Source: CAD feature listing. Evaluate the final solid. Frame: model axes, mm. Face numbers are marked on the shaded views. A direction names the side the tool comes from. Give positions to 0.01 mm unless a question says otherwise; leave off trailing zeros. Loops run counter-clockwise (first coordinate to the right, second up) from the corner with the lowest first, then second, coordinate; pieces in that order, holes last.
```python
from build123d import *

# Parameters (mm, degrees)
SKETCH_234_R           = 1.55
EXTRUDE_1_DEPTH        = 2.75
SKETCH_923_W           = 10.000000002
SKETCH_923_H           = 4.75
EXTRUDE_2_DEPTH        = 2.75
SKETCH_1070_W          = 1
SKETCH_1070_H          = 6.95
EXTRUDE_1769_DEPTH     = 2.75
PCB_START              = -4
SKETCH_6_W             = 1
SKETCH_6_H             = 6.95
PCB_DEPTH              = 4
SKETCH_4_W             = 1.75
SKETCH_4_H             = 28.99988509
CUT_EXTRUDE_2211_DEPTH = 1.5
SKETCH_5_W             = 0.25
SKETCH_5_H             = 28.99988509
CUT_EXTRUDE_2_DEPTH    = 33.350081892
CHAMFER_1_SIZE         = 1
CHAMFER_2_SIZE         = 1
CUT_EXTRUDE_4_DEPTH    = 4


with BuildPart() as part:
    # Sketch 234 → 底座-1 (new body)
    with BuildSketch(Plane(origin=(0, 0, 0), x_dir=(1, 0, 0), z_dir=(0, 1, 0))):
        with BuildLine():
            Line((22.500000002, -14.24988509), (22.500000002, -7.263629174))
            Line((22.500000002, -7.263629174), (24.500000002, -7.263629174))
            Line((24.500000002, -7.263629174), (24.500000002, 0.312480077))
            Line((24.500000002, 0.312480077), (24.715186194, 2.08073674))
            ThreePointArc((24.715186194, 2.08073674), (20.15501929, 5.688743466), (16.252981126, 10))
            Line((16.252981126, 10), (12.5, 10))
            Line((12.5, 10), (12.5, -14.24988509))
            Line((12.5, -14.24988509), (22.500000002, -14.24988509))
        make_face()
        with Locations(Location((16.865979255, 0, 0), (0, 0, 270))):
            Circle(SKETCH_234_R, mode=Mode.SUBTRACT)
    extrude(amount=EXTRUDE_1_DEPTH)

    # Sketch 923 → 底座-2 (add)
    with BuildSketch(Plane(origin=(0, 0, 0), x_dir=(1, 0, 0), z_dir=(0, 1, 0))):
        with Locations((17.500000001, -16.62488509)):
            Rectangle(SKETCH_923_W, SKETCH_923_H)
    extrude(amount=EXTRUDE_2_DEPTH)

    # Sketch 1070 → Extrude 1769 (add)
    with BuildSketch(Plane(origin=(0, 0, 0), x_dir=(1, 0, 0), z_dir=(0, 1, 0))):
        with BuildLine():
            ThreePointArc((24.715186194, 2.08073674), (25.291636518, 1.705823535), (25.875319612, 1.342273079))
            Line((25.875319612, 1.342273079), (25.750000002, 0.312480077))
            Line((25.750000002, 0.312480077), (25.750000002, -14.213629174))
            Line((25.750000002, -14.213629174), (24.500000002, -14.213629174))
            Line((24.500000002, -14.213629174), (24.500000002, -7.263629174))
            Line((24.500000002, -7.263629174), (24.500000002, 0.312480077))
            Line((24.500000002, 0.312480077), (24.715186194, 2.08073674))
        make_face()
        with Locations((24.000000002, -10.738629174)):
            Rectangle(SKETCH_1070_W, SKETCH_1070_H)
        with Locations((23.000000002, -10.738629174)):
            Rectangle(SKETCH_1070_W, SKETCH_1070_H)
    extrude(amount=EXTRUDE_1769_DEPTH)

    # Sketch 6 → 底座卡榫-注意PCB突出部分 (add)
    with BuildSketch(Plane(origin=(0, 0, 0), x_dir=(1, 0, 0), z_dir=(0, 1, 0)).offset(PCB_START)):
        with Locations((24.000000002, -10.738629174)):
            Rectangle(SKETCH_6_W, SKETCH_6_H)
        with BuildLine():
            ThreePointArc((24.715186194, 2.08073674), (25.291636518, 1.705823535), (25.875319612, 1.342273079))
            Line((25.875319612, 1.342273079), (25.750000002, 0.312480077))
            Line((25.750000002, 0.312480077), (25.750000002, -14.213629174))
            Line((25.750000002, -14.213629174), (24.500000002, -14.213629174))
            Line((24.500000002, -14.213629174), (24.500000002, -7.263629174))
            Line((24.500000002, -7.263629174), (24.500000002, 0.312480077))
            Line((24.500000002, 0.312480077), (24.715186194, 2.08073674))
        make_face()
    extrude(amount=PCB_DEPTH)

    # 草图4 → Cut-Extrude 2211 (cut)
    with BuildSketch(Plane(origin=(0, 0, 0), x_dir=(1, 0, 0), z_dir=(0, 1, 0))):
        with Locations((13.375, -4.499942545)):
            Rectangle(SKETCH_4_W, SKETCH_4_H)
    extrude(amount=CUT_EXTRUDE_2211_DEPTH, mode=Mode.SUBTRACT)

    # 草图5 → 配合切除-2 (cut, through all)
    with BuildSketch(Plane(origin=(0, 0, 0), x_dir=(1, 0, 0), z_dir=(0, 1, 0))):
        with Locations((12.625, -4.499942545)):
            Rectangle(SKETCH_5_W, SKETCH_5_H)
    extrude(amount=CUT_EXTRUDE_2_DEPTH, mode=Mode.SUBTRACT)

    # 倒角1
    chamfer_1_edges = [part.edges().sort_by_distance(p)[0] for p in [
        (22.500000002, 1.375, 18.99988509),
        (20.661675073, 2.75, -5.223818951),
        (22.500000002, 1.375, 14.213629174),
    ]]
    chamfer(chamfer_1_edges, length=CHAMFER_1_SIZE)

    # 倒角2
    chamfer_2_edges = [part.edges().sort_by_distance(p)[0] for p in [
        (16.865979255, 2.75, -1.55),
    ]]
    chamfer(chamfer_2_edges, length=CHAMFER_2_SIZE)

    # Sketch 6 2 → 切除-拉伸4 (cut)
    with BuildSketch(Plane.XZ.offset(4)):
        with BuildLine():
            Line((24.715186194, -2.08073674), (24.500000002, -0.312480077))
            Line((24.500000002, -0.312480077), (24.500000002, 7.263629174))
            Line((24.500000002, 7.263629174), (23.500000002, 7.263629174))
            Line((23.500000002, 7.263629174), (23.500000002, 7.513629174))
            Line((23.500000002, 7.513629174), (24.750000002, 7.513629174))
            Line((24.750000002, 7.513629174), (24.750000002, -0.312480077))
            Line((24.750000002, -0.312480077), (24.946632534, -1.928275128))
            ThreePointArc((24.946632534, -1.928275128), (24.830758909, -2.004277534), (24.715186194, -2.08073674))
        make_face()
    extrude(amount=-CUT_EXTRUDE_4_DEPTH, mode=Mode.SUBTRACT)


solid = part.part
```
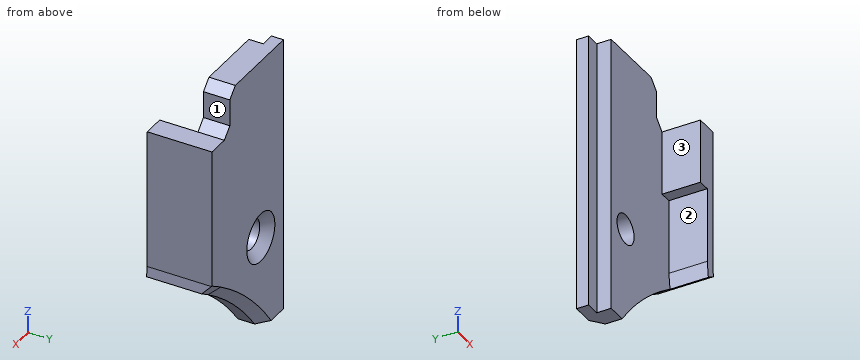
(1) Section C-C, the plane y = 1. Return the cut outline in (x, z), then the cut area to 3 significant figures.
A:
outline: (14.25, -10) - (16.25, -10) arc R35.11 cw to (24.72, -2.08) arc R35.11 cw to (25.88, -1.34) - (25.75, -0.31) - (25.75, 14.21) - (23.5, 14.21) - (22.5, 15.21) - (22.5, 18) - (21.5, 19) - (14.25, 19) - close; hole circle Ø3.1 at (16.87, 0)
area: 265 mm2
(2) First-contact query: pin 1 (0.7 mm diameter, centred on x = 24.5, y = -1.5, fed in from +Z); pin 2 (2 mm diameter, centred on y = -2.5, z = 10, fed in from -X); pin 3 (1 mm diameter, centred on x = 16.5, z = 9.5, fed in from -Y). Flat tips, straight axial feed; report the tip coordinate or a pass-through.
A:
pin 1: stops at z = 14.21
pin 2: stops at x = 23.5
pin 3: stops at y = 0
(3) Section A-A, the plane y = -2. Return the cut outline in (x, z), then the cut area to 3 significant figures.
A:
outline: (23.5, 7.51) - (24.75, 7.51) - (24.75, -0.31) - (24.95, -1.93) arc R35.11 cw to (25.88, -1.34) - (25.75, -0.31) - (25.75, 14.21) - (23.5, 14.21) - close
area: 24.2 mm2
(4) Ray query, line 1 along X through (y, z) = (1.2, 0); line 2 along Y through (x, z) = (22, 3.75); line 3 along Z through (x, y) = (23.75, -2.25). Return the intervals inside material, ascending.
A:
line 1: x = 14.25 to 15.32, 18.42 to 25.75
line 2: y = 0 to 2.75
line 3: z = 7.51 to 14.21
(5) Section B-B, the plane z = 11. Return the cut outline in (x, y), then the cut area to 3 significant figures.
A:
outline: (12.75, 1.5) - (14.25, 1.5) - (14.25, 0) - (23.5, 0) - (23.5, -4) - (25.75, -4) - (25.75, 2.75) - (12.75, 2.75) - close
area: 42.5 mm2
(6) Reachability of the marked faces 1, 2 and 3 from +Z, -Z, +X, -X, +Y, -Y: full face, straight path, thin tool, end or side. Return the list, or none.
A:
face 1: +Z, +X, +Y, -Y
face 2: -Z, -X, -Y
face 3: +Z, -Z, -X, -Y
